from build123d import *

# Parameters (mm, degrees)
BOSS_EXTRUDE1_DEPTH = 52


with BuildPart() as part:
    # Sketch2 → Boss-Extrude1 (new body)
    with BuildSketch(Plane.XY):
        with BuildLine():
            Line((0, 0), (24, 0))
            Line((24, 0), (24, 7.7))
            ThreePointArc((24, 7.7), (22.974873734, 10.174873734), (20.5, 11.2))
            Line((20.5, 11.2), (3.5, 11.2))
            ThreePointArc((3.5, 11.2), (1.025126266, 10.174873734), (0, 7.7))
            Line((0, 7.7), (0, 0))
        make_face()
    extrude(amount=BOSS_EXTRUDE1_DEPTH)


solid = part.part
Input: part model. Units: mm. Frame: model coordinates. Coordinates: 2 decimals unless noted, no trailing zeros. Order: outer loops, then holes, each group sorted by start corner. A loop starts at its lowest first (then second) coordinate and runs counter-clockwise, first axis right, second up. Notation, with made-up numbers: M 61.5,58.25 L 79.5,58.25 A31 cw 79.5,91.25 Z; hole C 31.5,-36 d10. An arc over 180 degrees is marked long. Answer as CSV lines item,"result".
1. Section A-A (z = 43.5). Return the cut outline in (x, y).
Reported:
outline,"M 0,0 L 24,0 L 24,7.7 A3.5 ccw 20.5,11.2 L 3.5,11.2 A3.5 ccw 0,7.7 Z"
2. Material intervals for line 1 (Y direction, x = 2, z = 40); line 2 (X direction, y = 9.75, z = 10.5); line 3 (Y direction, x = 1.75, z = 25), sorted ascending. Write a range as from..to.
Reported:
line 1,"0..10.86"
line 2,"0.66..23.34"
line 3,"0..10.73"
3. Pull-direction query (Z, two-part tool) for faces 1 (the flat face through (12, 6, 0)), 2 (the flat face through (12, 6, 52)), 3 (the cylindrical face through (1.05, 10.2, 25.64)); classes: released by +Z, released by -Z, zero draft, split by the parting line, or undercut.
Reported:
face 1,"released by -Z"
face 2,"released by +Z"
face 3,"zero draft"
